Geometry check sheet. Reference: the model listing, model coordinates, mm. Face numbers are marked on the shaded views. A direction names the side the tool comes from. Give positions to 0.01 mm unless a question says otherwise; leave off trailing zeros. Write each loop counter-clockwise with the first axis right and the second up, starting at its lowest first coordinate (ties: lowest second). Pieces come first, ordered by that corner, then holes. Notation, with made-up numbers: M 52.25,38.5 L 62.25,38.5 A25 cw 62.25,55.5 Z; hole C 30,66 d8. An arc over 180 degrees is marked long. One line per item, written item: value. Start each with the question number.
1. Gauge pin test, flat ends, axial feed: pin 1 (4 mm diameter, centred on x = 7, z = -25, fed in from +Y); pin 2 (10 mm diameter, centred on y = -1.5, z = -25.5, fed in from -X); pin 3 (5 mm diameter, centred on x = 9.5, z = -25, fed in from -Y). Record the tip position at first contact, or that the pin passes through.
2. Tool access check on the marked faces 4, 5, 6, 7 and 8. Record the directions out of +Z, -Z, +X, -X, +Y, -Y that give a thin tool (end or side, any length) a straight path to the whole face; none if there is none.
3. Cross-section at A-A on z = -4.5. Record the cut outline in (x, y).
4. Cross-section at B-B on y = 4.25. Record the cut outline in (x, z).
5. Scan lines: line 1 (X direction, y = -8, z = -6); line 2 (Y direction, x = -6.5, z = -9.5); line 3 (Y direction, x = 6.75, z = -16). Record each from-to range of solid material in increasing order.
6. Release check for a two-part mould opening along Y. For the marked faces 1, 2 and 3 record: pulls with the +Y half, pulls with the -Y half, needs draft (parallel to the pull), parting line crosses it, or undercut.
7. Cross-section at C-C on x = 0. Record the cut outline in (y, z).
8. Cross-section at D-D on z = -8.5. Record the cut outline in (x, y).
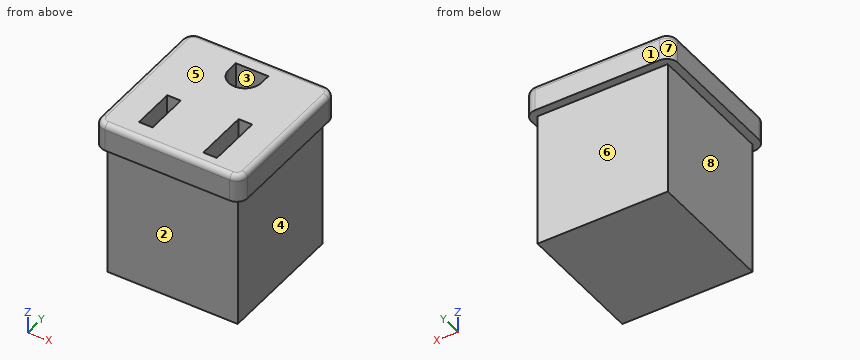
Autodesk Inventor part; units mm, degrees
ref_plane "YZ Plane" through (0, 0, 0) normal (1, 0, 0) x (0, 1, 0)
ref_plane "XZ Plane" through (0, 0, 0) normal (0, 1, 0) x (-1, 0, 0)
ref_plane "XY Plane" through (0, 0, 0) normal (0, 0, 1) x (1, 0, 0)
sketch "Sketch1" plane through (0, 0, 0) normal (0, 0, 1) x (1, 0, 0)
  line L0 (-13.5, 13.5) -> (13.5, 13.5)
  line L1 (13.5, 13.5) -> (13.5, -13.5)
  line L2 (13.5, -13.5) -> (-13.5, -13.5)
  line L3 (-13.5, -13.5) -> (-13.5, 13.5)
  point P0 (0, 0)
  dimension "d0" = 27
  dimension "d2" = 27
  dimension "d3" = 13.5
  dimension "d4" = 13.5
extrude "Extrusion1" add sketch "Sketch1" against normal blind 5
sketch "Sketch2" plane through (0, 0, -5) normal (0, 0, -1) x (-1, 0, 0)
  line L0 (13.5, 13.5) -> (-13.5, 13.5)
  line L1 (-13.5, 13.5) -> (-13.5, -13.5)
  line L2 (-12, 12) -> (12, 12)
  line L3 (12, 12) -> (12, -12)
  line L4 (12, -12) -> (-12, -12)
  line L5 (-12, -12) -> (-12, 12)
  point P0 (0, 0)
  dimension "d7" = 24
  dimension "d8" = 24
  dimension "d9" = 1.5
  dimension "d10" = 1.5
extrude "Extrusion2" add sketch "Sketch2" along normal blind 25
sketch "Sketch3" plane through (0, 0, 0) normal (0, 0, 1) x (1, 0, 0)
  line L0 (-13.5, 13.5) -> (13.5, 13.5)
  line L1 (13.5, 13.5) -> (13.5, -13.5)
  line L2 (-3, 10.5) -> (3, 10.5)
  line L3 (3, 10.5) -> (3, 8.5)
  line L4 (-3, 10.5) -> (-3, 8.5)
  arc A0 (-3, 8.5) -> (3, 8.5) centre (0, 8.5) ccw
  line L5 (-7.5, -2) -> (-5, -2)
  line L6 (-5, -2) -> (-5, -10)
  line L7 (-5, -10) -> (-7.5, -10)
  line L8 (-7.5, -10) -> (-7.5, -2)
  line L9 (5, -1) -> (7.5, -1)
  line L10 (7.5, -1) -> (7.5, -11)
  line L11 (7.5, -11) -> (5, -11)
  line L12 (5, -11) -> (5, -1)
  point P0 (0, 0)
  dimension "d13" = 6
  dimension "d15" = 2
  dimension "d18" = 0
  dimension "d19" = 3
  dimension "d20" = 2.5
  dimension "d21" = 2.5
  dimension "d22" = 10
  dimension "d23" = 8
  dimension "d24" = 5
  dimension "d25" = 5
  dimension "d26" = 1
  dimension "d27" = 2
extrude "Extrusion3" cut sketch "Sketch3" against normal blind 20
fillet "Fillet1" radius 2 4 edges at (13.5, 13.5, -2.5) (13.5, -13.5, -2.5) (-13.5, -13.5, -2.5) (-13.5, 13.5, -2.5)
fillet "Fillet2" radius 1 8 edges at (12.9142, -12.9142, 0) (0, -13.5, 0) (-12.9142, -12.9142, 0) (-13.5, 0, 0) (-12.9142, 12.9142, 0) (0, 13.5, 0) (12.9142, 12.9142, 0) (13.5, 0, 0)
properties part number "739W-X203"
Report:
1. pin 1: stops at y = 12
1. pin 2: stops at x = -12
1. pin 3: stops at y = -12
2. face 4: -Z, +X, +Y, -Y
2. face 5: +Z, +X, -X, +Y, -Y
2. face 6: -Z, +X, -X, +Y
2. face 7: +Z, -Z, -X, +Y
2. face 8: -Z, -X, +Y, -Y
3. outline: M -13.5,-11.5 A2 ccw -11.5,-13.5 L 11.5,-13.5 A2 ccw 13.5,-11.5 L 13.5,11.5 A2 ccw 11.5,13.5 L -11.5,13.5 A2 ccw -13.5,11.5 Z; hole M -7.5,-10 L -5,-10 L -5,-2 L -7.5,-2 Z; hole M -3,8.5 A3 ccw 3,8.5 L 3,10.5 L -3,10.5 Z; hole M 5,-11 L 7.5,-11 L 7.5,-1 L 5,-1 Z
4. outline: M -13.5,-5 L -12,-5 L -12,-30 L 12,-30 L 12,-5 L 13.5,-5 L 13.5,-1 A1 ccw 12.5,0 L -12.5,0 A1 ccw -13.5,-1 Z
5. line 1: x = -12 to -7.5, -5 to 5, 7.5 to 12
5. line 2: y = -12 to -10, -2 to 12
5. line 3: y = -12 to -11, -1 to 12
6. face 1: pulls with the +Y half
6. face 2: pulls with the -Y half
6. face 3: undercut
7. outline: M -13.5,-5 L -12,-5 L -12,-30 L 12,-30 L 12,-5 L 13.5,-5 L 13.5,-1 A1 ccw 12.5,0 L 10.5,0 L 10.5,-20 L 5.5,-20 L 5.5,0 L -12.5,0 A1 ccw -13.5,-1 Z
8. outline: M -12,-12 L 12,-12 L 12,12 L -12,12 Z; hole M -7.5,-10 L -5,-10 L -5,-2 L -7.5,-2 Z; hole M -3,8.5 A3 ccw 3,8.5 L 3,10.5 L -3,10.5 Z; hole M 5,-11 L 7.5,-11 L 7.5,-1 L 5,-1 Z
